```python
from build123d import *

# Parameters (mm, degrees)
SKETCH1_W           = 25
SKETCH1_H           = 24
SKETCH1_R           = 1
BOSS_EXTRUDE1_DEPTH = 1
SKETCH2_W           = 8
SKETCH2_H           = 8
BOSS_EXTRUDE2_DEPTH = 4
SKETCH3_R           = 4
BOSS_EXTRUDE3_DEPTH = 1
FILLET2_R           = 0.5
SKETCH4_W           = 16
SKETCH4_H           = 5
BOSS_EXTRUDE4_DEPTH = 2
FILLET3_R           = 0.5
SKETCH5_R           = 3.5
CUT_EXTRUDE1_DEPTH  = 6
BOSS_EXTRUDE5_DEPTH = 1
SKETCH7_W           = 0.2
SKETCH7_H           = 4.34
CUT_EXTRUDE2_DEPTH  = 1
LPATTERN1_COUNT     = 14
LPATTERN1_PITCH     = 0.3
SKETCH8_W           = 15
SKETCH8_H           = 1
BOSS_EXTRUDE6_DEPTH = 20


with BuildPart() as part:
    # Sketch1 → Boss-Extrude1 (new body)
    with BuildSketch(Plane.XY):
        Rectangle(SKETCH1_W, SKETCH1_H)
        with Locations((10.5, 10)):
            Circle(SKETCH1_R, mode=Mode.SUBTRACT)
        with Locations((-10.5, 10)):
            Circle(SKETCH1_R, mode=Mode.SUBTRACT)
        with Locations((-10.5, -2.5)):
            Circle(SKETCH1_R, mode=Mode.SUBTRACT)
        with Locations((10.5, -2.5)):
            Circle(SKETCH1_R, mode=Mode.SUBTRACT)
    extrude(amount=BOSS_EXTRUDE1_DEPTH)

    # Sketch2 → Boss-Extrude2 (add)
    with BuildSketch(Plane.XY.offset(1)):
        with Locations((0, -2.5)):
            Rectangle(SKETCH2_W, SKETCH2_H)
    extrude(amount=BOSS_EXTRUDE2_DEPTH)

    # Sketch3 → Boss-Extrude3 (add)
    with BuildSketch(Plane.XY.offset(5)):
        with Locations((0, -2.5)):
            Circle(SKETCH3_R)
    extrude(amount=BOSS_EXTRUDE3_DEPTH)

    # Fillet2
    fillet2_edges = [part.edges().sort_by_distance(p)[0] for p in [
        (4, -2.5, 1),
        (-4, -2.5, 1),
        (0, -6.5, 1),
    ]]
    fillet(fillet2_edges, radius=FILLET2_R)

    # Sketch4 → Boss-Extrude4 (add)
    with BuildSketch(Plane(origin=(0, 0, 0), x_dir=(-1, 0, 0), z_dir=(0, 0, -1))):
        with Locations((0, -7.5)):
            Rectangle(SKETCH4_W, SKETCH4_H)
    extrude(amount=BOSS_EXTRUDE4_DEPTH)

    # Fillet3
    fillet3_edges = [part.edges().sort_by_distance(p)[0] for p in [
        (-8, -7.5, 0),
        (-8, -10, -1),
        (0, -5, 0),
        (-8, -5, -1),
        (8, -7.5, 0),
        (8, -5, -1),
        (0, -10, 0),
        (8, -10, -1),
        (-8, -7.5, -2),
        (0, -5, -2),
        (8, -7.5, -2),
        (0, -10, -2),
    ]]
    fillet(fillet3_edges, radius=FILLET3_R)

    # Sketch5 → Cut-Extrude1 (cut)
    with BuildSketch(Plane.XY.offset(6)):
        with Locations((0, -2.5)):
            Circle(SKETCH5_R)
    extrude(amount=-CUT_EXTRUDE1_DEPTH, mode=Mode.SUBTRACT)

    # Sketch6 → Boss-Extrude5 (add)
    with BuildSketch(Plane.XY.offset(1)):
        Polygon((-3.152517362, 10.68), (-3.152517362, 5.84), (-2.322578899, 5.84), (-2.322578899, 1.5), (2.017421101, 1.5), (2.017421101, 5.84), (2.846354447, 5.84), (2.846354447, 6.468877905), (2.846354447, 10.68), align=None)
    extrude(amount=BOSS_EXTRUDE5_DEPTH)

    # Sketch7 → Cut-Extrude2 (cut)
    with BuildSketch(Plane.XY.offset(2)):
        with Locations((-2.072578899, 3.67)):
            Rectangle(SKETCH7_W, SKETCH7_H)
    cut_extrude2 = extrude(amount=-CUT_EXTRUDE2_DEPTH, mode=Mode.SUBTRACT)

    # LPattern1: Cut-Extrude2 ×14
    with Locations(*[(i * LPATTERN1_PITCH, 0, 0) for i in range(1, LPATTERN1_COUNT)]):
        add(cut_extrude2, mode=Mode.SUBTRACT)

    # Sketch8 → Boss-Extrude6 (add)
    with BuildSketch(Plane.XZ.offset(10)):
        with Locations((0, -1)):
            Rectangle(SKETCH8_W, SKETCH8_H)
    extrude(amount=BOSS_EXTRUDE6_DEPTH)


solid = part.part
```
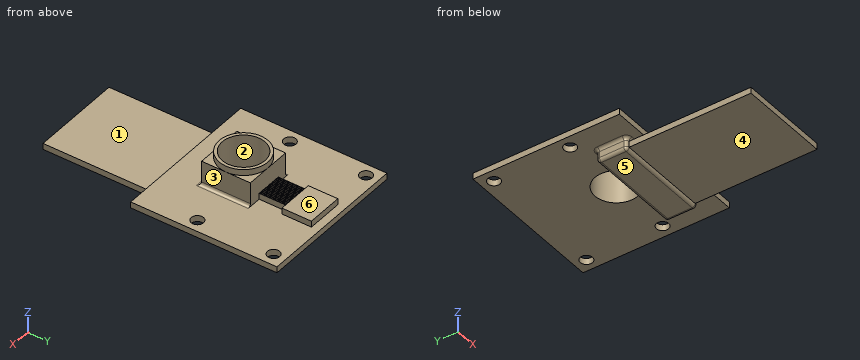
Input: part model. Units: mm. Frame: model coordinates. Face numbers are marked on the shaded views. A direction names the side the tool comes from. Give positions to 0.01 mm unless a question says otherwise; leave off trailing zeros. Order: outer loops, then holes, each group sorted by start corner. A loop starts at its lowest first (then second) coordinate and runs counter-clockwise, first axis right, second up. Notation, with made-up numbers: (4.25, -5.75) -> (56.25, -5.75) arc R22 cw to (56.25, 1.25) -> close; hole circle Ø5 at (-34.5, -37.5). An arc over 180 degrees is marked (long way). Write each question's results on one line, items separated by ' | '. Start each with the question number.
Item 1: Set-up query: the marked faces 3, 4, 5 and 6. Return all of +Z, -Z, +X, -X, +Y, -Y with unobstructed straight access to the full face (end or side cutting, diameter ignored); none if empty.
Item 2: Line query: line 1 (Y direction, x = 10.5, z = 0.3); line 2 (X direction, y = -2.5, z = 2.75); line 3 (Y direction, x = 0, z = 3.5). Output: solid intervals per line, ascending.
Item 3: Cut plane C-C on y = -15. Return the cut outline in (x, z).
Item 4: Cut plane A-A on y = 10. Return the cut outline in (x, z), then the cut area to 3 significant figures.
Item 5: Contact query for flat-ended pins moving along their axis: P1, Ø1.1, axis at x = -1.5, z = 1.5, coming from the +Y side; P2, Ø1.5, axis at x = 3, z = 2, coming from the +Y side; P3, Ø2, axis at x = -2, z = 4, coming from the -Y side; P4, Ø0.8, axis at y = -7.5, z = -1, coming from the -X side. Output: stop coordinate, or through.
Item 6: Cut plane B-B on x = -10.5. Return the cut outline in (y, z), then the cut area to 3 significant figures.
Item 7: Mould query, pull axis Y, two halves, no side actions, for the marked faces 1 and 2. Classes: pulls with the +Y half, pulls with the -Y half, needs draft (parallel to the pull), parting line crosses it, or undercut.
Item 8: Cut plane D-D on x = 10.25. Return the cut outline in (y, z), then the cut area to 3 significant figures.
Established:
1) face 3: +Z, +X, +Y, -Y | face 4: -Z, +X, -X, -Y | face 5: -Z, +X, -X, +Y, -Y | face 6: +Z, +X, -X, +Y
2) line 1: -12 to -3.5, -1.5 to 9, 11 to 12 | line 2: -4 to -3.5, 3.5 to 4 | line 3: -6.5 to -6, 1 to 1.5
3) outline: (-7.5, -1.5) -> (7.5, -1.5) -> (7.5, -0.5) -> (-7.5, -0.5) -> close
4) outline: (-12.5, 0) -> (-11.5, 0) -> (-11.5, 1) -> (-12.5, 1) -> close; (-9.5, 0) -> (9.5, 0) -> (9.5, 1) -> (2.85, 1) -> (2.85, 2) -> (-3.15, 2) -> (-3.15, 1) -> (-9.5, 1) -> close; (11.5, 0) -> (12.5, 0) -> (12.5, 1) -> (11.5, 1) -> close | area: 27.0 mm^2
5) P1: y = 12 | P2: y = 10.68 | P3: y = -6.5 | P4: x = -8
6) outline: (-12, 0) -> (-3.5, 0) -> (-3.5, 1) -> (-12, 1) -> close; (-1.5, 0) -> (9, 0) -> (9, 1) -> (-1.5, 1) -> close; (11, 0) -> (12, 0) -> (12, 1) -> (11, 1) -> close | area: 20.0 mm^2
7) face 1: needs draft | face 2: undercut
8) outline: (-12, 0) -> (-3.47, 0) -> (-3.47, 1) -> (-12, 1) -> close; (-1.53, 0) -> (9.03, 0) -> (9.03, 1) -> (-1.53, 1) -> close; (10.97, 0) -> (12, 0) -> (12, 1) -> (10.97, 1) -> close | area: 20.1 mm^2
